Read the model definition and answer for the solid it produces. Units are mm, in the model's axes. Coordinates: 2 decimals unless noted, no trailing zeros. Loops run counter-clockwise (first coordinate to the right, second up) from the corner with the lowest first, then second, coordinate; pieces in that order, holes last. Notation, with made-up numbers: (45, 63.25) - (58, 63.25) arc R21 ccw to (58, 77.25) - close; hole circle Ø5 at (50.5, 83.25). An arc over 180 degrees is marked (long way). Use CSV: the item, a comma, the result in double quotes.
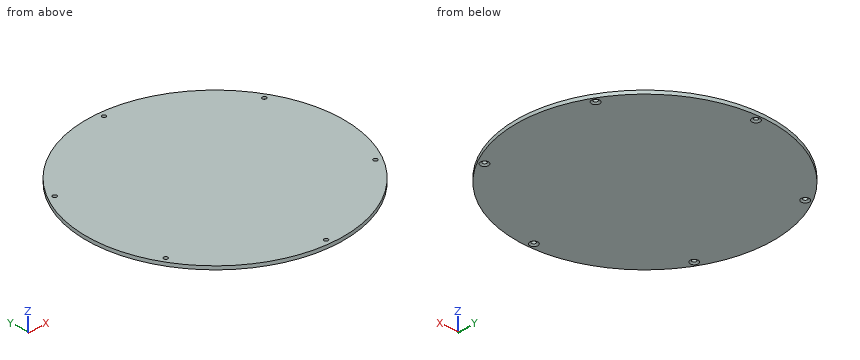
```python
from build123d import *
from OCP.BRepFilletAPI import BRepFilletAPI_MakeChamfer

# Parameters (mm, degrees)
CROQUIS1_R              = 110
CROQUIS1_R_2            = 1.75
SALIENTE_EXTRUIR1_DEPTH = 3
CHAFL_N1_SIZE           = 1
CHAFL_N1_SIZE2          = 1.732050808
CHAFL_N2_SIZE           = 1
CHAFL_N2_SIZE2          = 1.732050808


with BuildPart() as part:
    # Croquis1 → Saliente-Extruir1 (new body)
    with BuildSketch(Plane.XY):
        Circle(CROQUIS1_R)
        with Locations((0, 105)):
            Circle(CROQUIS1_R_2, mode=Mode.SUBTRACT)
        with Locations((90.932667397, 52.5)):
            Circle(CROQUIS1_R_2, mode=Mode.SUBTRACT)
        with Locations((90.932667397, -52.5)):
            Circle(CROQUIS1_R_2, mode=Mode.SUBTRACT)
        with Locations((0, -105)):
            Circle(CROQUIS1_R_2, mode=Mode.SUBTRACT)
        with Locations((-90.932667397, -52.5)):
            Circle(CROQUIS1_R_2, mode=Mode.SUBTRACT)
        with Locations((-90.932667397, 52.5)):
            Circle(CROQUIS1_R_2, mode=Mode.SUBTRACT)
    extrude(amount=SALIENTE_EXTRUIR1_DEPTH)

    # Chaflán1
    chafl_n1_edges = [part.edges().sort_by_distance(p)[0] for p in [
        (-1.75, 105, 0),
    ]]
    chafl_n1_side = [part.faces().sort_by_distance(p)[0] for p in [
        (-1.75, 105, 1.5),
    ]]
    chamfer(chafl_n1_edges, length=CHAFL_N1_SIZE, length2=CHAFL_N1_SIZE2, reference=chafl_n1_side[0])

    # Chaflán2: one chamfer whose edges measure the first distance from different faces: ONE call of the kernel's chamfer builder (chamfer() names one face for all edges)
    chafl_n2_edges_1 = [part.edges().sort_by_distance(p)[0] for p in [
        (89.182667397, -52.5, 0),
    ]]
    chafl_n2_side_1 = [part.faces().sort_by_distance(p)[0] for p in [
        (89.182667397, -52.5, 1.5),
    ]]
    chafl_n2_edges_2 = [part.edges().sort_by_distance(p)[0] for p in [
        (-1.75, -105, 0),
    ]]
    chafl_n2_side_2 = [part.faces().sort_by_distance(p)[0] for p in [
        (-1.75, -105, 1.5),
    ]]
    chafl_n2_edges_3 = [part.edges().sort_by_distance(p)[0] for p in [
        (-92.682667397, -52.5, 0),
    ]]
    chafl_n2_side_3 = [part.faces().sort_by_distance(p)[0] for p in [
        (-92.682667397, -52.5, 1.5),
    ]]
    chafl_n2_edges_4 = [part.edges().sort_by_distance(p)[0] for p in [
        (-92.682667397, 52.5, 0),
    ]]
    chafl_n2_side_4 = [part.faces().sort_by_distance(p)[0] for p in [
        (-92.682667397, 52.5, 1.5),
    ]]
    chafl_n2_edges_5 = [part.edges().sort_by_distance(p)[0] for p in [
        (89.182667397, 52.5, 0),
    ]]
    chafl_n2_side_5 = [part.faces().sort_by_distance(p)[0] for p in [
        (89.182667397, 52.5, 1.5),
    ]]
    chafl_n2 = BRepFilletAPI_MakeChamfer(part.part.solid().wrapped)
    for e in chafl_n2_edges_1:
        chafl_n2.Add(CHAFL_N2_SIZE, CHAFL_N2_SIZE2, e.wrapped, chafl_n2_side_1[0].wrapped)  # the first distance lies on this face
    for e in chafl_n2_edges_2:
        chafl_n2.Add(CHAFL_N2_SIZE, CHAFL_N2_SIZE2, e.wrapped, chafl_n2_side_2[0].wrapped)  # the first distance lies on this face
    for e in chafl_n2_edges_3:
        chafl_n2.Add(CHAFL_N2_SIZE, CHAFL_N2_SIZE2, e.wrapped, chafl_n2_side_3[0].wrapped)  # the first distance lies on this face
    for e in chafl_n2_edges_4:
        chafl_n2.Add(CHAFL_N2_SIZE, CHAFL_N2_SIZE2, e.wrapped, chafl_n2_side_4[0].wrapped)  # the first distance lies on this face
    for e in chafl_n2_edges_5:
        chafl_n2.Add(CHAFL_N2_SIZE, CHAFL_N2_SIZE2, e.wrapped, chafl_n2_side_5[0].wrapped)  # the first distance lies on this face
    add(Compound.cast(chafl_n2.Shape()), mode=Mode.REPLACE)


solid = part.part
```
Q1. The part is cut by section A-A on z = 1.8. Determine the outline of the cut face in (x, y).
Reported:
outline,"circle Ø220 at (0, 0); hole circle Ø3.5 at (-90.93, -52.5); hole circle Ø3.5 at (-90.93, 52.5); hole circle Ø3.5 at (0, -105); hole circle Ø3.5 at (0, 105); hole circle Ø3.5 at (90.93, -52.5); hole circle Ø3.5 at (90.93, 52.5)"
Q2. Find the intervals of material crossed by probe 1 along Y at (x, z) = (90, 2.5); probe 2 along X at (y, z) = (-52, 2.4); probe 3 along X at (y, z) = (53, 2.2), in increasing order. Write a range as [from, to].
Reported:
probe 1,"y = [-63.25, -53.98], [-51.02, 51.02], [53.98, 63.25]"
probe 2,"x = [-96.93, -92.61], [-89.26, 89.26], [92.61, 96.93]"
probe 3,"x = [-96.39, -92.61], [-89.26, 89.26], [92.61, 96.39]"
Q3. Given P1, Ø8, axis at x = -11.5, y = 64, coming from the -Z side; P2, Ø5.5, axis at x = 90.93, y = -52.5, coming from the -Z side; P3, Ø4.5, axis at x = -90.93, y = -52.5, coming from the -Z side; P4, Ø4, axis at x = -90.93, y = 52.5, coming from the -Z side, each flat-ended and moving along its own axis, determine where each tip first touches the part or whether it passes through.
Reported:
P1,"stops at z = 0"
P2,"stops at z = 0.42"
P3,"stops at z = 0.71"
P4,"stops at z = 0.85"
Q4. The part is cut by section B-B on x = -66. Determine the outline of the cut face in (y, z), and give its area (3 significant figures).
Reported:
outline,"(-88, 0) - (88, 0) - (88, 3) - (-88, 3) - close"
area,"528 mm²"
Q5. The part is cut by section C-C on x = 37. Determine the outline of the cut face in (y, z).
Reported:
outline,"(-103.59, 0) - (103.59, 0) - (103.59, 3) - (-103.59, 3) - close"
